Can you work these out from the model? Positions are in its coordinate system, mm. Face numbers are marked on the shaded views. A direction names the side the tool comes from. Give positions to 0.01 mm unless a question says otherwise; leave off trailing zeros. Write each loop counter-clockwise with the first axis right and the second up, starting at its lowest first coordinate (ties: lowest second). Pieces come first, ordered by that corner, then holes. Notation, with made-up numbers: (65.5, 6) - (93.5, 6) arc R28 cw to (93.5, 28) - close; hole circle Ø7 at (38, -17.75). An arc over 180 degrees is marked (long way). Use a Markdown table: item, result. Add a question column.
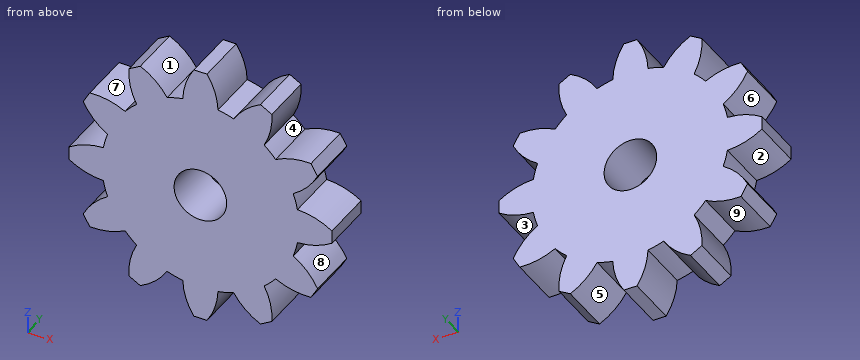
```python
from build123d import *

# Parameters (mm, degrees)
SKETCH1_R           = 4
BOSS_EXTRUDE1_DEPTH = 4


with BuildPart() as part:
    # Sketch1 → Boss-Extrude1 (new body, symmetric)
    with BuildSketch(Plane(origin=(0, 0, 0), x_dir=(1, 0, 0), z_dir=(0, 1, 0))):
        with BuildLine():
            Line((-1, 20), (1, 20))
            ThreePointArc((1, 20), (2.204975942, 17.497232023), (2.675, 14.759551992))
            ThreePointArc((2.675, 14.759551992), (3.882285677, 14.488887394), (5.063158041, 14.119646973))
            ThreePointArc((5.063158041, 14.119646973), (6.839050831, 16.255535399), (9.133974596, 17.820508076))
            Line((9.133974596, 17.820508076), (10.866025404, 16.820508076))
            ThreePointArc((10.866025404, 16.820508076), (10.658181192, 14.050559457), (9.696393951, 11.444646973))
            ThreePointArc((9.696393951, 11.444646973), (10.606601718, 10.606601718), (11.444646973, 9.696393951))
            ThreePointArc((11.444646973, 9.696393951), (14.050559457, 10.658181192), (16.820508076, 10.866025404))
            Line((16.820508076, 10.866025404), (17.820508076, 9.133974596))
            ThreePointArc((17.820508076, 9.133974596), (16.255535399, 6.839050831), (14.119646973, 5.063158041))
            ThreePointArc((14.119646973, 5.063158041), (14.488887394, 3.882285677), (14.759551992, 2.675))
            ThreePointArc((14.759551992, 2.675), (17.497232023, 2.204975942), (20, 1))
            Line((20, 1), (20, -1))
            ThreePointArc((20, -1), (17.497232023, -2.204975942), (14.759551992, -2.675))
            ThreePointArc((14.759551992, -2.675), (14.488887394, -3.882285677), (14.119646973, -5.063158041))
            ThreePointArc((14.119646973, -5.063158041), (16.255535399, -6.839050831), (17.820508076, -9.133974596))
            Line((17.820508076, -9.133974596), (16.820508076, -10.866025404))
            ThreePointArc((16.820508076, -10.866025404), (14.050559457, -10.658181192), (11.444646973, -9.696393951))
            ThreePointArc((11.444646973, -9.696393951), (10.606601718, -10.606601718), (9.696393951, -11.444646973))
            ThreePointArc((9.696393951, -11.444646973), (10.658181192, -14.050559457), (10.866025404, -16.820508076))
            Line((10.866025404, -16.820508076), (9.133974596, -17.820508076))
            ThreePointArc((9.133974596, -17.820508076), (6.839050831, -16.255535399), (5.063158041, -14.119646973))
            ThreePointArc((5.063158041, -14.119646973), (3.882285677, -14.488887394), (2.675, -14.759551992))
            ThreePointArc((2.675, -14.759551992), (2.204975942, -17.497232023), (1, -20))
            Line((1, -20), (-1, -20))
            ThreePointArc((-1, -20), (-2.204975942, -17.497232023), (-2.675, -14.759551992))
            ThreePointArc((-2.675, -14.759551992), (-3.882285677, -14.488887394), (-5.063158041, -14.119646973))
            ThreePointArc((-5.063158041, -14.119646973), (-6.839050831, -16.255535399), (-9.133974596, -17.820508076))
            Line((-9.133974596, -17.820508076), (-10.866025404, -16.820508076))
            ThreePointArc((-10.866025404, -16.820508076), (-10.658181192, -14.050559457), (-9.696393951, -11.444646973))
            ThreePointArc((-9.696393951, -11.444646973), (-10.606601718, -10.606601718), (-11.444646973, -9.696393951))
            ThreePointArc((-11.444646973, -9.696393951), (-14.050559457, -10.658181192), (-16.820508076, -10.866025404))
            Line((-16.820508076, -10.866025404), (-17.820508076, -9.133974596))
            ThreePointArc((-17.820508076, -9.133974596), (-16.255535399, -6.839050831), (-14.119646973, -5.063158041))
            ThreePointArc((-14.119646973, -5.063158041), (-14.488887394, -3.882285677), (-14.759551992, -2.675))
            ThreePointArc((-14.759551992, -2.675), (-17.497232023, -2.204975942), (-20, -1))
            Line((-20, -1), (-20, 1))
            ThreePointArc((-20, 1), (-17.497232023, 2.204975942), (-14.759551992, 2.675))
            ThreePointArc((-14.759551992, 2.675), (-14.488887394, 3.882285677), (-14.119646973, 5.063158041))
            ThreePointArc((-14.119646973, 5.063158041), (-16.255535399, 6.839050831), (-17.820508076, 9.133974596))
            Line((-17.820508076, 9.133974596), (-16.820508076, 10.866025404))
            ThreePointArc((-16.820508076, 10.866025404), (-14.050559457, 10.658181192), (-11.444646973, 9.696393951))
            ThreePointArc((-11.444646973, 9.696393951), (-10.606601718, 10.606601718), (-9.696393951, 11.444646973))
            ThreePointArc((-9.696393951, 11.444646973), (-10.658181192, 14.050559457), (-10.866025404, 16.820508076))
            Line((-10.866025404, 16.820508076), (-9.133974596, 17.820508076))
            ThreePointArc((-9.133974596, 17.820508076), (-6.839050831, 16.255535399), (-5.063158041, 14.119646973))
            ThreePointArc((-5.063158041, 14.119646973), (-3.882285677, 14.488887394), (-2.675, 14.759551992))
            ThreePointArc((-2.675, 14.759551992), (-2.204975942, 17.497232023), (-1, 20))
        make_face()
        Circle(SKETCH1_R, mode=Mode.SUBTRACT)
    extrude(amount=BOSS_EXTRUDE1_DEPTH, both=True)


solid = part.part
```
Q1. Suppose I cut it at C-C (x = 16). Please give me the cut outline in (y, z).
Q2. Suppose I cut it at B-B (z = 0). Please give me the cut outline in (x, y).
Q3. Suppose I cut it at D-D (x = -13). Please give me the cut outline in (y, z).
Q4. If we mould it in two halves opening along X, with no side actions, what happens to the marked faces 6, 7, 8 and 9? For each: released by +X, released by -X, zero draft, split by the parting line, or undercut.
Q5. On a 3-axis mill with a long thin cutter (end or side, diameter ignored), from which of +Z, -Z, +X, -X, +Y, -Y can I reach the whole of each face in a straight line? I mean the marked faces 1, 2, 3, 4 and 5. Say none if no direction works.
Q6. If I drill on probe 1 along X at (y, z) = (2.5, 0); probe 2 along X at (y, z) = (-3.5, -17.5), over which ranges is the centre line in solid material (lowest first)? Write a range as [from, to].
Q7. I'm going to push flat-ended pins straight in: P1, Ø1, axis at y = -0.5, z = -14.5, coming from the -X side; P2, Ø3, axis at y = 0, z = -12.5, coming from the -X side. Where does each tip first touch, or does it pass through?
Q8. Suppose I cut it at A-A (x = 0). Please give me the cut outline in (y, z), and give its area (3 significant figures).
Derived:
| question | item | result |
|---|---|---|
| 1 | outline | (-4, -10.89) - (4, -10.89) - (4, -6.57) - (-4, -6.57) - close; (-4, -2.56) - (4, -2.56) - (4, 2.56) - (-4, 2.56) - close; (-4, 6.57) - (4, 6.57) - (4, 10.89) - (-4, 10.89) - close |
| 2 | outline | (-20, -4) - (-4, -4) - (-4, 4) - (-20, 4) - close; (4, -4) - (20, -4) - (20, 4) - (4, 4) - close |
| 3 | outline | (-4, -10.37) - (4, -10.37) - (4, 10.37) - (-4, 10.37) - close |
| 4 | face 6 | released by -X |
| 4 | face 7 | undercut |
| 4 | face 8 | released by +X |
| 4 | face 9 | undercut |
| 5 | face 1 | +Z, +Y, -Y |
| 5 | face 2 | -X, +Y, -Y |
| 5 | face 3 | +X, +Y, -Y |
| 5 | face 4 | +Y, -Y |
| 5 | face 5 | -Z, +Y, -Y |
| 6 | probe 1 | [-20, -4], [4, 20] |
| 6 | probe 2 | [-9.69, -8.54], [-2.2, 2.2], [8.54, 9.69] |
| 7 | P1 | x = -10.82 |
| 7 | P2 | x = -10.65 |
| 8 | outline | (-4, -20) - (4, -20) - (4, -4) - (-4, -4) - close; (-4, 4) - (4, 4) - (4, 20) - (-4, 20) - close |
| 8 | area | 256 mm² |
